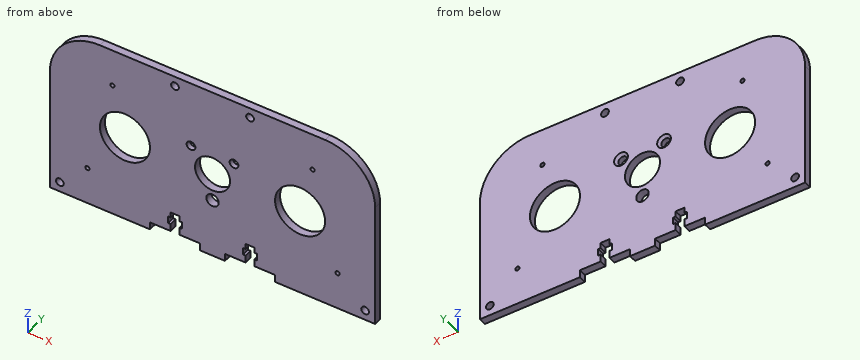
Solid Edge part; units mm, degrees
sketch "Sketch1" plane through (0, 0, 0) normal (0, -1, 0) x (1, 0, 0)
  line L0 (-65, -35) -> (65, -35)
  line L1 (65, -35) -> (65, 35)
  line L2 (65, 35) -> (-65, 35)
  line L3 (-65, 35) -> (-65, -35)
  dimension "D1" = 65
  dimension "D2" = 65
extrude "Ajout_matière_1" add sketch "Sketch1" along normal blind 3
sketch "Sketch2" plane through (0, -3, 0) normal (0, -1, 0) x (1, 0, 0)
  circle A0 centre (35, 0) radius 10
extrude "Enlèvement_matière_1" cut sketch "Sketch2" against normal blind 203.2796
sketch "Sketch3" plane through (0, -3, 0) normal (0, -1, 0) x (1, 0, 0)
  circle A0 centre (40, 20) radius 0.85
  circle A1 centre (15, 31) radius 1.55
  circle A2 centre (61, -31) radius 1.55
  circle A3 centre (50, -20) radius 0.85
  circle A4 centre (8.6, 8.29) radius 1.75
  dimension "D1" = 40
  dimension "D2" = 50
extrude "Enlèvement_matière_2" cut sketch "Sketch3" against normal blind 33.5111
sketch "Sketch4" plane through (0, -3, 0) normal (0, -1, 0) x (1, 0, 0)
  line L0 (5, -38) -> (25, -38)
  line L1 (25, -38) -> (25, -32)
  line L2 (16.75, -32) -> (25, -32)
  line L3 (16.75, -29) -> (16.75, -32)
  line L4 (17.77, -29) -> (16.75, -29)
  line L5 (17.77, -26.2) -> (17.77, -29)
  line L6 (16.75, -26.2) -> (17.77, -26.2)
  line L7 (16.75, -24) -> (16.75, -26.2)
  line L8 (13.25, -24) -> (16.75, -24)
  line L9 (13.25, -26.2) -> (13.25, -24)
  line L10 (12.23, -26.2) -> (13.25, -26.2)
  line L11 (12.23, -29) -> (12.23, -26.2)
  line L12 (13.25, -29) -> (12.23, -29)
  line L13 (13.25, -32) -> (13.25, -29)
  line L14 (5, -32) -> (13.25, -32)
  line L15 (5, -32) -> (5, -38)
  dimension "D1" = 5
  dimension "D2" = 5
  dimension "D3" = 5
  dimension "D4" = 13.25
  dimension "D5" = 13.25
  dimension "D6" = 5
  dimension "D7" = 12.23
extrude "Cutout1" cut sketch "Sketch4" against normal blind 6.6007
mirror "Mirror1" about plane through (0, 0, 0) normal (1, 0, 0) of "Enlèvement_matière_1", "Enlèvement_matière_2", "Cutout1"
fillet "Congé_1" radius 20 1 edges at (65, -1.5, 35)
fillet "Round1" radius 20 1 edges at (-65, -1.5, 35)
sketch "Sketch5" plane through (0, -3, 0) normal (0, -1, 0) x (1, 0, 0)
  circle A0 centre (0, 0) radius 7
  circle A1 centre (0, -11.25) radius 2.5
extrude "Enlèvement_matière_8" cut sketch "Sketch5" against normal blind 3.6745
chamfer "Chamfer1" distance 1 angle 45 2 edges at (-8.6, 0, 10.04) (8.6, 0, 10.04)
properties part number "07" material "MDF 3mm"
Geometry check sheet. Reference: the model listing, model coordinates, mm. Give positions to 0.01 mm unless a question says otherwise; leave off trailing zeros. Order: outer loops, then holes, each group sorted by start corner. A loop starts at its lowest first (then second) coordinate and runs counter-clockwise, first axis right, second up.
1) Material ranges on probe 1 along X at (y, z) = (-0.1, 0.5); probe 2 along Z at (x, y) = (-15, -1.55); probe 3 along X at (y, z) = (-1.95, -4), recorded low to high.
Results are:
probe 1: x = -65 to -44.99, -25.01 to -6.98, 6.98 to 25.01, 44.99 to 65
probe 2: z = -24 to 29.45, 32.55 to 35
probe 3: x = -65 to -44.17, -25.83 to -5.74, 5.74 to 25.83, 44.17 to 65
2) Gauge pin test, flat ends, axial feed: pin 1 (12 mm diameter, centred on x = -35, z = 0, fed in from -Y); pin 2 (16 mm diameter, centred on x = 0, z = 0, fed in from -Y); pin 3 (1.5 mm diameter, centred on x = 15, y = -2, fed in from -Z); pin 4 (4 mm diameter, centred on x = -8.6, z = 8.29, fed in from +Y). Record the tip position at first contact, or that the pin passes through.
Results are:
pin 1: passes through
pin 2: stops at y = -3
pin 3: stops at z = -24
pin 4: stops at y = -0.75
3) Cross-section at D-D (z = 31). Record the boundary of the cut face in (x, y), then the cut area to 3 significant figures.
Results are:
outline: (-57, -3) - (-16.55, -3) - (-16.55, 0) - (-57, 0) - close; (-13.45, -3) - (13.45, -3) - (13.45, 0) - (-13.45, 0) - close; (16.55, -3) - (57, -3) - (57, 0) - (16.55, 0) - close
area: 323 mm2
4) Cross-section at B-B (z = -11.25). Record the boundary of the cut face in (x, y), then the cut area to 3 significant figures.
Results are:
outline: (-65, -3) - (-2.5, -3) - (-2.5, 0) - (-65, 0) - close; (2.5, -3) - (65, -3) - (65, 0) - (2.5, 0) - close
area: 375 mm2
5) Cross-section at C-C (z = 0). Record the boundary of the cut face in (x, y).
Results are:
outline: (-65, -3) - (-45, -3) - (-45, 0) - (-65, 0) - close; (-25, -3) - (-7, -3) - (-7, 0) - (-25, 0) - close; (7, -3) - (25, -3) - (25, 0) - (7, 0) - close; (45, -3) - (65, -3) - (65, 0) - (45, 0) - close
6) Cross-section at A-A (x = 35). Record the boundary of the cut face in (y, z), then the cut area to 3 significant figures.
Results are:
outline: (-3, -35) - (0, -35) - (0, -10) - (-3, -10) - close; (-3, 10) - (0, 10) - (0, 35) - (-3, 35) - close
area: 150 mm2
